```python
from build123d import *

# Parameters (mm, degrees)
F0_W     = 67.4
F0_H     = 43
F1_DEPTH = 1.7
F2_R     = 1.55
F3_DEPTH = 25
F4_W     = 25.107336
F4_H     = 9.729092
F4_W_2   = 17.339753
F4_H_2   = 9.179869
F5_DEPTH = 8.6
F4_R     = 3.25
F6_DEPTH = 12
F4_W_3   = 20.085868
F4_H_3   = 2.353814
F4_H_4   = 2.353812
F7_DEPTH = 8.4
F4_W_4   = 7.061438
F4_H_5   = 17.231865
F8_DEPTH = 5.8


with BuildPart() as f1:
    # F0 (on Top) → F1 (new body)
    with BuildSketch(Plane.XY):
        Rectangle(F0_W, F0_H)
    extrude(amount=F1_DEPTH)

    # F2 (on face) → F3 (cut)
    with BuildSketch(Plane.XY.offset(1.7)):
        with Locations((-29.85, 18.15)):
            Circle(F2_R)
        with Locations((3.15, -17.55)):
            Circle(F2_R)
        with Locations((30.55, 18.05)):
            Circle(F2_R)
    extrude(amount=-F3_DEPTH, mode=Mode.SUBTRACT)

    # F4 (on face) → F5 (join)
    with BuildSketch(Plane.XY.offset(1.7)):
        with Locations((-10.797692, -3.640961)):
            Rectangle(F4_W, F4_H)
        with Locations((18.507275, -1.169458)):
            Rectangle(F4_W_2, F4_H_2)
    extrude(amount=F5_DEPTH)

    # F4 (on face) → F6 (join)
    with BuildSketch(Plane.XY.offset(1.7)):
        with Locations((7.008187, -13.818246)):
            Circle(F4_R)
        with Locations((7.008187, 11.673535)):
            Circle(F4_R)
        with Locations((29.902235, 11.673535)):
            Circle(F4_R)
        with Locations((29.902235, -13.818246)):
            Circle(F4_R)
    extrude(amount=F6_DEPTH)

    # F4 (on face) → F7 (join)
    with BuildSketch(Plane.XY.offset(1.7)):
        with Locations((-10.797692, -18.940743)):
            Rectangle(F4_W_3, F4_H_3)
        with Locations((17.134217, 19.269482)):
            Rectangle(F4_W_3, F4_H_4)
    extrude(amount=F7_DEPTH)

    # F4 (on face) → F8 (join)
    with BuildSketch(Plane.XY.offset(1.7)):
        with Locations((-5.697765, 11.673535)):
            Rectangle(F4_W_4, F4_H_5)
    extrude(amount=F8_DEPTH)


solid = f1.part
```
Geometry check sheet. Reference: the model listing, model coordinates, mm. A direction names the side the tool comes from. Give positions to 0.01 mm unless a question says otherwise; leave off trailing zeros. Loops run counter-clockwise (first coordinate to the right, second up) from the corner with the lowest first, then second, coordinate; pieces in that order, holes last. Notation, with made-up numbers: M 31.25,44 L 51.25,44 A19 cw 51.25,76 Z; hole C 58.5,22.5 d1. An arc over 180 degrees is marked long. Write item = value, one per line. Start each with the question number.
1. Go/stop test with flat-tipped pins: P1, Ø2, axis at x = 21.5, y = 11.5, coming from the +Z side; P2, Ø4, axis at x = 14.5, z = 9, coming from the +Y side; P3, Ø2.5, axis at x = 16, y = 19, coming from the +Z side; P4, Ø6, axis at x = 13, y = -14.5, coming from the +Z side. Record where each tip stops, or that it passes through.
2. Draft check along Y on faces 6 (the face through (17, 19, 10.1)), 7 (the face through (31.4, 8.79, 7.62)), 8 (the face through (17, 20.446, 6)). Enter one of: +Y half, -Y half, draft (parallel to the pull), parting line (faces both ways), or undercut.
3. Section check A-A, the plane x = -29.85. Enter the section's corners in (y, z), plus the area to 3 significant figures.
4. Thickness scan on probe 1 along Y at (x, z) = (3.15, 1.05); probe 2 along Y at (x, z) = (-1, 8); probe 3 along X at (y, z) = (14, 2). Record the ranges inside material, lowest first.
5. Tool access check on faces 1 (the face through (-20.841, -19, 6)), 2 (the face through (-9.228, 12, 5)), 3 (the face through (1.756, -4, 6)), 4 (the face through (-11, -17.764, 6)), 5 (the face through (-6, 3.058, 5)). Record the directions out of +Z, -Z, +X, -X, +Y, -Y that give a thin tool (end or side, any length) a straight path to the whole face; none if there is none.
6. Section check B-B, the plane x = 26. Enter the section's corners in (y, z), plus the area to 3 significant figures.
7. Section check D-D, the plane y = -4.5. Enter the section's corners in (x, z).
8. Section check C-C, the plane z = 4. Give the number of separate pieces and of enclosed holes in the cut face, plus the area to 3 significant figures.
Values follow:
q1.P1 = 1.7
q1.P2 = 20.45
q1.P3 = 10.1
q1.P4 = 13.7
q2.face_6 = draft
q2.face_7 = undercut
q2.face_8 = +Y half
q3.outline = M -21.5,0 L 16.6,0 L 16.6,1.7 L -21.5,1.7 Z; M 19.7,0 L 21.5,0 L 21.5,1.7 L 19.7,1.7 Z
q3.area = 67.8 mm^2
q4.probe_1 = -21.5 to -19.1, -16 to 21.5
q4.probe_2 = -20.12 to -17.76, -8.51 to 1.22
q4.probe_3 = -9.23 to -2.17, 4.74 to 9.28, 27.63 to 32.17
q5.face_1 = +Z, -X, -Y
q5.face_2 = +Z, -X, +Y
q5.face_3 = +Z, +Y, -Y
q5.face_4 = +Z, +X, -X
q5.face_5 = +Z, -X
q6.outline = M -21.5,0 L 21.5,0 L 21.5,1.7 L 20.45,1.7 L 20.45,10.1 L 18.09,10.1 L 18.09,1.7 L 3.42,1.7 L 3.42,10.3 L -5.76,10.3 L -5.76,1.7 L -21.5,1.7 Z
q6.area = 172 mm^2
q7.outline = M -33.7,0 L 33.7,0 L 33.7,1.7 L 27.18,1.7 L 27.18,10.3 L 9.84,10.3 L 9.84,1.7 L 1.76,1.7 L 1.76,10.3 L -23.35,10.3 L -23.35,1.7 L -33.7,1.7 Z
q8.separate_pieces = 9
q8.enclosed_holes = 0
q8.area = 752 mm^2
